Geometry check sheet. Reference: the model listing, model coordinates, mm. A direction names the side the tool comes from. Round coordinates to 2 decimals unless told otherwise and drop trailing zeros. Loops run counter-clockwise (first coordinate to the right, second up) from the corner with the lowest first, then second, coordinate; pieces in that order, holes last. Notation, with made-up numbers: (49, 83.25) - (68, 83.25) arc R28 ccw to (68, 102.25) - close; hole circle Ø11 at (50, -13). An arc over 180 degrees is marked (long way). Write item = value, one per line.
```python
from build123d import *

# Parameters (mm, degrees)
SKETCH1_W           = 17
SKETCH1_H           = 12
SKETCH1_H_2         = 42
SKETCH1_H_3         = 34
SKETCH1_H_4         = 18
SKETCH1_H_5         = 20
BOSS_EXTRUDE1_DEPTH = 5


with BuildPart() as part:
    # Sketch1 → Boss-Extrude1 (new body)
    with BuildSketch(Plane(origin=(0, 0, 0), x_dir=(1, 0, 0), z_dir=(0, 1, 0))):
        Polygon((-58.5, 30), (-58.5, -30), (-51.975, -30), (-51.975, -18.45), (51.975, -18.45), (51.975, -30), (58.5, -30), (58.5, 30), align=None)
        with Locations((22, -1)):
            Rectangle(SKETCH1_W, SKETCH1_H, mode=Mode.SUBTRACT)
        with Locations((-44, 6)):
            Rectangle(SKETCH1_W, SKETCH1_H_2, mode=Mode.SUBTRACT)
        with Locations((-22, 10)):
            Rectangle(SKETCH1_W, SKETCH1_H_3, mode=Mode.SUBTRACT)
        with Locations((0, 10)):
            Rectangle(SKETCH1_W, SKETCH1_H_3, mode=Mode.SUBTRACT)
        with Locations((22, 18)):
            Rectangle(SKETCH1_W, SKETCH1_H_4, mode=Mode.SUBTRACT)
        with Locations((44, 17)):
            Rectangle(SKETCH1_W, SKETCH1_H_5, mode=Mode.SUBTRACT)
    extrude(amount=BOSS_EXTRUDE1_DEPTH)


solid = part.part
```
(1) Mould release check, pull along Z, two halves, no side actions. Record for faces 3 (the flat face through (-51.975, 2, 24)), 4 (the flat face through (55, 2, 30)), 5 (the flat face through (52.5, 2, -17)): pulls with the +Z half, pulls with the -Z half, needs draft (parallel to the pull), parting line crosses it, or undercut.
Answers follow:
face_3 = needs draft
face_4 = pulls with the +Z half
face_5 = undercut
(2) Section check D-D (x = 2.5). Enter the section's corners in (y, z).
Answers follow:
outline = (0, -30) - (5, -30) - (5, -27) - (0, -27) - close; (0, 7) - (5, 7) - (5, 18.45) - (0, 18.45) - close
(3) Section check C-C (z = 23). Enter the section's corners in (x, y) (3 decimals).
Answers follow:
outline = (-58.5, 0) - (-51.975, 0) - (-51.975, 5) - (-58.5, 5) - close; (51.975, 0) - (58.5, 0) - (58.5, 5) - (51.975, 5) - close
(4) Section check A-A (z = 4). Enter the section's corners in (x, y).
Answers follow:
outline = (-58.5, 0) - (-52.5, 0) - (-52.5, 5) - (-58.5, 5) - close; (-35.5, 0) - (-30.5, 0) - (-30.5, 5) - (-35.5, 5) - close; (-13.5, 0) - (-8.5, 0) - (-8.5, 5) - (-13.5, 5) - close; (8.5, 0) - (13.5, 0) - (13.5, 5) - (8.5, 5) - close; (30.5, 0) - (58.5, 0) - (58.5, 5) - (30.5, 5) - close
(5) Scan lines: L1, parallel to X at y = 1.05, z = -14.5; L2, parallel to Z at x = 20.5, y = 4.3; L3, parallel to X at y = 4.75, z = 1.5. Record each from-to range of solid material in increasing order. Write a range as [from, to].
Answers follow:
L1 = [-58.5, -52.5], [-35.5, -30.5], [-13.5, -8.5], [8.5, 13.5], [30.5, 35.5], [52.5, 58.5]
L2 = [-30, -27], [-9, -5], [7, 18.45]
L3 = [-58.5, -52.5], [-35.5, -30.5], [-13.5, -8.5], [8.5, 13.5], [30.5, 58.5]
(6) Set-up check for faces 1 (the flat face through (58.5, 2, 0)), 2 (the flat face through (35.5, 2, -17)): record each of +Z, -Z, +X, -X, +Y, -Y from which the full face is reachable in a straight line by a thin tool's end or side.
Answers follow:
face_1 = +Z, -Z, +X, +Y, -Y
face_2 = +Y, -Y
(7) Gauge pin test, flat end, axial feed: pin 1 (1.5 mm diameter, centred on x = 18, y = 3.5, fed in from +Z). Record the tip position at first contact, or that the pin passes through.
Answers follow:
pin_1 = 18.45
(8) Section check B-B (y = 3.4). State how many separate pieces and enclosed holes the cut face has, then the cut area to 3 significant figures.
Answers follow:
separate_pieces = 1
enclosed_holes = 6
area = 3,100 mm²
